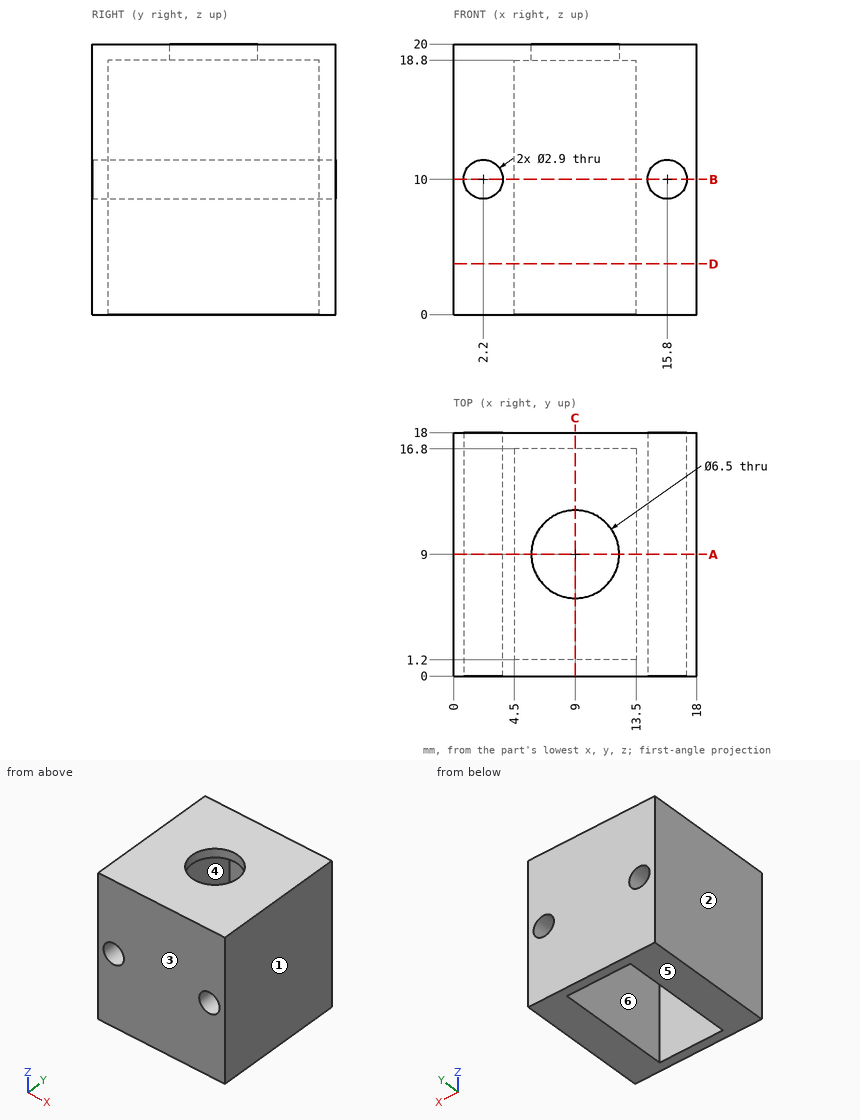
Job drawing, mm, ordinate dimensions from the low corner. One solid piece. A direction names the side the tool comes from. Coordinates: 2 decimals unless noted, no trailing zeros. Write each loop counter-clockwise with the first axis right and the second up, starting at its lowest first coordinate (ties: lowest second). Pieces come first, ordered by that corner, then holes. Notation, with made-up numbers: M -7.75,72 L -3.75,72 A11 cw -3.75,76 Z; hole C -18.75,60 d7. An arc over 180 degrees is marked long. Answer as a JSON object with one key per item and string values. Group by question number.
1) Saw through at A-A (y = 9). Write the cut outline in (x, z), plus the area to 3 significant figures.
2) Saw through at C-C (x = 9). Write the cut outline in (y, z), plus the area to 3 significant figures.
3) Saw through at B-B (z = 10). Write the cut outline in (x, y), plus the area to 3 significant figures.
4) Tool access for the marked faces 5 and 6: list every direction of +Z, -Z, +X, -X, +Y, -Y with a clear straight run to the whole face (end or side of a thin tool).
5) Wall check: line 1 (X direction, y = 14, z = 12); line 2 (Z direction, x = 2.2, y = 9); line 3 (Y direction, x = 8, z = 3.5). Give the ranges that are in metal, low to high. Write a range as from..to.
6) Saw through at D-D (z = 3.75). Write the cut outline in (x, y).
7) Pin check, flat tips, straight feed: pin 1 Ø2.5 at (x, y) = (7.5, 8.5) entering from -Z; pin 2 Ø5 at (x, y) = (10.5, 4.5) entering from -Z. Stop position of each tip, or through.
8) Mould opens along X. For the marked faces 1, 2, 3 and 4 say: +X half, -X half, draft (parallel to the pull), parting line (faces both ways), or undercut.
Values follow:
{
 "1": {"outline": "M 0,0 L 4.5,0 L 4.5,18.8 L 5.75,18.8 L 5.75,20 L 0,20 Z; M 12.25,18.8 L 13.5,18.8 L 13.5,0 L 18,0 L 18,20 L 12.25,20 Z; hole C 2.2,10 d2.9; hole C 15.8,10 d2.9", "area": "170 mm2"},
 "2": {"outline": "M 0,0 L 1.2,0 L 1.2,18.8 L 5.75,18.8 L 5.75,20 L 0,20 Z; M 12.25,18.8 L 16.8,18.8 L 16.8,0 L 18,0 L 18,20 L 12.25,20 Z", "area": "58.9 mm2"},
 "3": {"outline": "M 0,0 L 0.75,0 L 0.75,18 L 0,18 Z; M 3.65,0 L 14.35,0 L 14.35,18 L 3.65,18 Z; M 17.25,0 L 18,0 L 18,18 L 17.25,18 Z; hole M 4.5,1.2 L 13.5,1.2 L 13.5,16.8 L 4.5,16.8 Z", "area": "79.2 mm2"},
 "4": {"face 5": "-Z, +X, -X, +Y, -Y", "face 6": "-Z"},
 "5": {"line 1": "x = 0..4.5, 13.5..18", "line 2": "z = 0..8.55, 11.45..20", "line 3": "y = 0..1.2, 16.8..18"},
 "6": {"outline": "M 0,0 L 18,0 L 18,18 L 0,18 Z; hole M 4.5,1.2 L 13.5,1.2 L 13.5,16.8 L 4.5,16.8 Z"},
 "7": {"pin 1": "passes through", "pin 2": "stops at z = 18.8"},
 "8": {"face 1": "+X half", "face 2": "-X half", "face 3": "draft", "face 4": "undercut"}
}
